Model file for the job. Use its own axes, mm. Give positions to 0.01 mm unless a question says otherwise; leave off trailing zeros. Write each loop counter-clockwise with the first axis right and the second up, starting at its lowest first coordinate (ties: lowest second). Pieces come first, ordered by that corner, then holes. Notation, with made-up numbers: M -32,63 L 18,63 A32 cw 18,94 Z; hole C -29.75,22.25 d9. An arc over 180 degrees is marked long. Answer as a JSON object with one key per item and string values. Group by question number.
```python
from build123d import *

# Parameters (mm, degrees)
BOSS_EXTRUDE2_DEPTH  = 609.6
CUT_EXTRUDE1_DEPTH   = 1016
M6_CLEARANCE_HOLE1_D = 6.4
BOSS_EXTRUDE3_DEPTH  = 254


with BuildPart() as part:
    # Sketch3 → Boss-Extrude2 (new, symmetric)
    with BuildSketch(Plane.XY):
        Polygon((-15.875, 12.7), (-15.875, -12.7), (15.875, -12.7), (15.875, 12.7), (12.7, 12.7), (12.7, -9.525), (-12.7, -9.525), (-12.7, 12.7), align=None)
    extrude(amount=BOSS_EXTRUDE2_DEPTH, both=True)

    # Sketch5 → Cut-Extrude1 (cut)
    with BuildSketch(Plane.XY.offset(609.6)):
        Polygon((-15.875, 12.7), (-12.7, 12.7), (-12.7, -9.525), (12.7, -9.525), (12.7, 12.7), (15.875, 12.7), (15.875, -12.7), (-15.875, -12.7), align=None)
    extrude(amount=-CUT_EXTRUDE1_DEPTH, mode=Mode.SUBTRACT)

    # M6 Clearance Hole1 (through all)
    with Locations(Plane(origin=(0, -9.525, 0), x_dir=(1, 0, 0), z_dir=(0, 1, 0))):
        with Locations((0, 594.6)):
            Hole(M6_CLEARANCE_HOLE1_D / 2)

    # Sketch8 → Boss-Extrude3 (add)
    with BuildSketch(Plane(origin=(0, 0, -609.6), x_dir=(-1, 0, 0), z_dir=(0, 0, -1))):
        Polygon((-15.875, 12.7), (-12.7, 12.7), (-12.7, -9.525), (12.7, -9.525), (12.7, 12.7), (15.875, 12.7), (15.875, -12.7), (-15.875, -12.7), align=None)
    extrude(amount=BOSS_EXTRUDE3_DEPTH)


solid = part.part
```
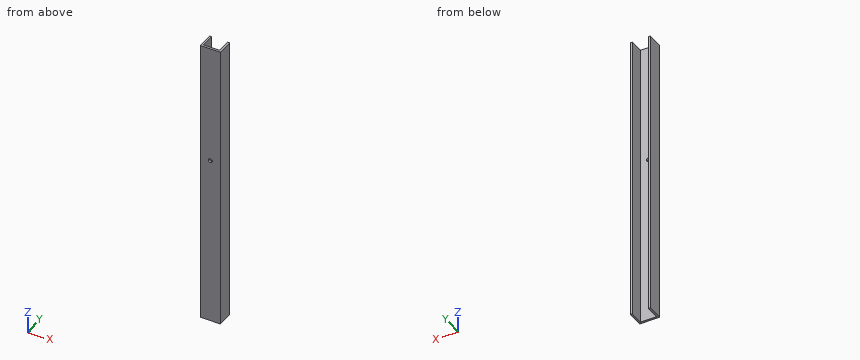
Q1. Slice it at A-A, the plane y = 0.25. Write the cut outline in (x, z) (3 decimals).
Q2. Drop flat-ended pins along their axis: P1, Ø6, axis at x = 0, z = -594.6, coming from the -Y side; P2, Ø3, axis at x = -6, z = -741, coming from the +Y side (3 decimals). Give the stop position or say it passes through.
Q3. Wall check: L1, parallel to X at y = 5, z = -647 (3 decimals); L2, parallel to X at y = -10.75, z = -594.6 (3 decimals); L3, parallel to Z at x = 0, y = -11.1. Give the ranges that are in metal, low to high.
Q4. Slice it at B-B, the plane z = -463. Write the cut outline in (x, y) (3 decimals).
Q5. Slice it at C-C, the plane x = 9. Write the cut outline in (y, z) (3 decimals), then the cut area to 3 significant figures.
Solved:
{
 "1": {"outline": "M -15.875,-863.6 L -12.7,-863.6 L -12.7,-406.4 L -15.875,-406.4 Z; M 12.7,-863.6 L 15.875,-863.6 L 15.875,-406.4 L 12.7,-406.4 Z"},
 "2": {"P1": "passes through", "P2": "stops at y = -9.525"},
 "3": {"L1": "x = -15.875 to -12.7, 12.7 to 15.875", "L2": "x = -15.875 to -3.2, 3.2 to 15.875", "L3": "z = -863.6 to -597.8, -591.4 to -406.4"},
 "4": {"outline": "M -15.875,-12.7 L 15.875,-12.7 L 15.875,12.7 L 12.7,12.7 L 12.7,-9.525 L -12.7,-9.525 L -12.7,12.7 L -15.875,12.7 Z"},
 "5": {"outline": "M -12.7,-863.6 L -9.525,-863.6 L -9.525,-406.4 L -12.7,-406.4 Z", "area": "1,450 mm²"}
}
